from build123d import *

# Parameters (mm, degrees)
SKETCH1_R           = 12.7
BOSS_EXTRUDE1_DEPTH = 8.6
FILLET2_R           = 0.75


with BuildPart() as part:
    # Sketch1 → Boss-Extrude1 (new body)
    with BuildSketch(Plane(origin=(0, 0, 0), x_dir=(1, 0, 0), z_dir=(0, 1, 0))):
        with BuildLine():
            Line((88.844407291, -2.475), (88.844407291, -7.400365603))
            ThreePointArc((88.844407291, -7.400365603), (93.263798172, 0), (88.844407291, 7.400365603))
            Line((88.844407291, 7.400365603), (88.844407291, 2.475))
            Line((88.844407291, 2.475), (87.144407291, 2.475))
            Line((87.144407291, 2.475), (87.144407291, 8.377664326))
            ThreePointArc((87.144407291, 8.377664326), (86.01145531, 8.60710798), (84.85806661, 8.684043601))
            Line((84.85806661, 8.684043601), (82.194407291, 8.684043601))
            Line((82.194407291, 8.684043601), (82.194407291, 2.475))
            Line((82.194407291, 2.475), (26.35, 2.475))
            Line((26.35, 2.475), (26.35, 7.425))
            Line((26.35, 7.425), (21.4, 7.425))
            Line((21.4, 7.425), (21.4, 2.475))
            Line((21.4, 2.475), (17.65, 2.475))
            Line((17.65, 2.475), (17.65, 17.65))
            Line((17.65, 17.65), (0, 17.65))
            ThreePointArc((0, 17.65), (-17.65, 0), (0, -17.65))
            Line((0, -17.65), (17.65, -17.65))
            Line((17.65, -17.65), (17.65, -2.475))
            Line((17.65, -2.475), (21.4, -2.475))
            Line((21.4, -2.475), (21.4, -7.425))
            Line((21.4, -7.425), (26.35, -7.425))
            Line((26.35, -7.425), (26.35, -2.475))
            Line((26.35, -2.475), (82.194407291, -2.475))
            Line((82.194407291, -2.475), (82.194407291, -8.684043601))
            Line((82.194407291, -8.684043601), (84.85806661, -8.684043601))
            ThreePointArc((84.85806661, -8.684043601), (86.01145531, -8.60710798), (87.144407291, -8.377664326))
            Line((87.144407291, -8.377664326), (87.144407291, -2.475))
            Line((87.144407291, -2.475), (88.844407291, -2.475))
        make_face()
        with Locations(Location((0, 0, 0), (0, 0, 90))):
            Circle(SKETCH1_R, mode=Mode.SUBTRACT)
    extrude(amount=BOSS_EXTRUDE1_DEPTH)

    # Fillet2
    fillet2_edges = [part.edges().sort_by_distance(p)[0] for p in [
        (21.4, 4.3, -7.425),
        (26.35, 4.3, -7.425),
        (82.194407291, 4.3, -2.475),
        (82.194407291, 4.3, -8.684043601),
        (87.144407291, 4.3, -8.377664326),
        (88.844407291, 4.3, -7.400365603),
        (88.844407291, 4.3, 7.400365603),
        (87.144407291, 4.3, 8.377664326),
        (82.194407291, 4.3, 8.684043601),
        (82.194407291, 4.3, 2.475),
        (26.35, 4.3, 7.425),
        (21.4, 4.3, 7.425),
        (17.65, 4.3, 17.65),
        (17.65, 4.3, -17.65),
    ]]
    fillet(fillet2_edges, radius=FILLET2_R)


solid = part.part
Can you work these out from the model? Positions are in its coordinate system, mm. A direction names the side the tool comes from. Coordinates: 2 decimals unless noted, no trailing zeros. Loops run counter-clockwise (first coordinate to the right, second up) from the corner with the lowest first, then second, coordinate; pieces in that order, holes last. Notation, with made-up numbers: (69.5, 10) - (85.5, 10) arc R15 cw to (85.5, 22) - close; hole circle Ø5 at (31.25, 4.25). An arc over 180 degrees is marked (long way). Put each result on its own line as item: value. Start each with the question number.
Item 1: Suppose I cut it at C-C (x = 66). Please give me the cut outline in (y, z) (3 decimals).
Item 2: If I drill on line 1 along X through (y, z) = (4.25, 0); line 2 along X through (y, z) = (8.25, -4.5); line 3 along X through (y, z) = (8, 7), over which ranges is the centre line in solid material (lowest first)?
Item 3: Suppose I cut it at A-A (z = 0). Please give me the cut outline in (x, y), and give its area (3 significant figures).
Item 4: For pin 1 (3.5 mm diameter, centred on y = 6.5, z = -4, fed in from -X); pin 2 (1.4 mm diameter, centred on x = 88, y = 3.5, fed in from +Z) (3 decimals); pin 3 (1.5 mm diameter, centred on y = 1, z = -6.5, fed in from +X); pin 4 (6 mm diameter, centred on x = 6, z = -6.5, fed in from +Y), each with a flat end and sliding along its axis, tell me the tip position at first contact or that it passes through.
Item 5: Suppose I cut it at D-D (z = -15). Please give me the cut outline in (x, y), and give its area (3 significant figures).
Item 6: Suppose I cut it at B-B (x = -2). Please give me the cut outline in (y, z), and give its area (3 significant figures).
Item 7: Which directions (+Z, -Z, +X, -X, +Y, -Y) give clear straight access to the entire face, cutting with the end or side of a thin tool? Please do faces 1 (the face through (24, 4, -7.425)), 2 (the face through (54, 4, 2.475)), 3 (the face through (-17.646, 4.24, -0.388)), 4 (the face through (84, 4, -8.684)).
Item 8: If we mould it in two halves opening along X, with no side actions, what happens to faces 5 (the face through (84, 4, 8.684)), 6 (the face through (87.144, 4, 5)), 7 (the face through (93.263, 4.24, 0.106))? For each: +X half, -X half, draft (parallel to the pull), parting line (faces both ways), or undercut.
Here are the results:
1. outline: (0, -2.475) - (8.6, -2.475) - (8.6, 2.475) - (0, 2.475) - close
2. line 1: -17.65 to -12.7, 12.7 to 93.26
2. line 2: -17.07 to -11.88, 11.88 to 17.65, 21.4 to 26.35, 82.19 to 87.14, 88.84 to 91.96
2. line 3: -16.2 to -10.6, 10.6 to 17.65, 21.47 to 26.28, 82.19 to 87.14
3. outline: (-17.65, 0) - (-12.7, 0) - (-12.7, 8.6) - (-17.65, 8.6) - close; (12.7, 0) - (93.26, 0) - (93.26, 8.6) - (12.7, 8.6) - close
3. area: 735 mm²
4. pin 1: x = -17.51
4. pin 2: z = 2.475
4. pin 3: x = 90.99
4. pin 4: through
5. outline: (-9.3, 0) - (17.65, 0) - (17.65, 8.6) - (-9.3, 8.6) - close
5. area: 232 mm²
6. outline: (0, -17.54) - (8.6, -17.54) - (8.6, -12.54) - (0, -12.54) - close; (0, 12.54) - (8.6, 12.54) - (8.6, 17.54) - (0, 17.54) - close
6. area: 85.9 mm²
7. face 1: -Z, +Y, -Y
7. face 2: +Z, +Y, -Y
7. face 3: -X, +Y, -Y
7. face 4: -Z, +X, +Y, -Y
8. face 5: draft
8. face 6: undercut
8. face 7: +X half
